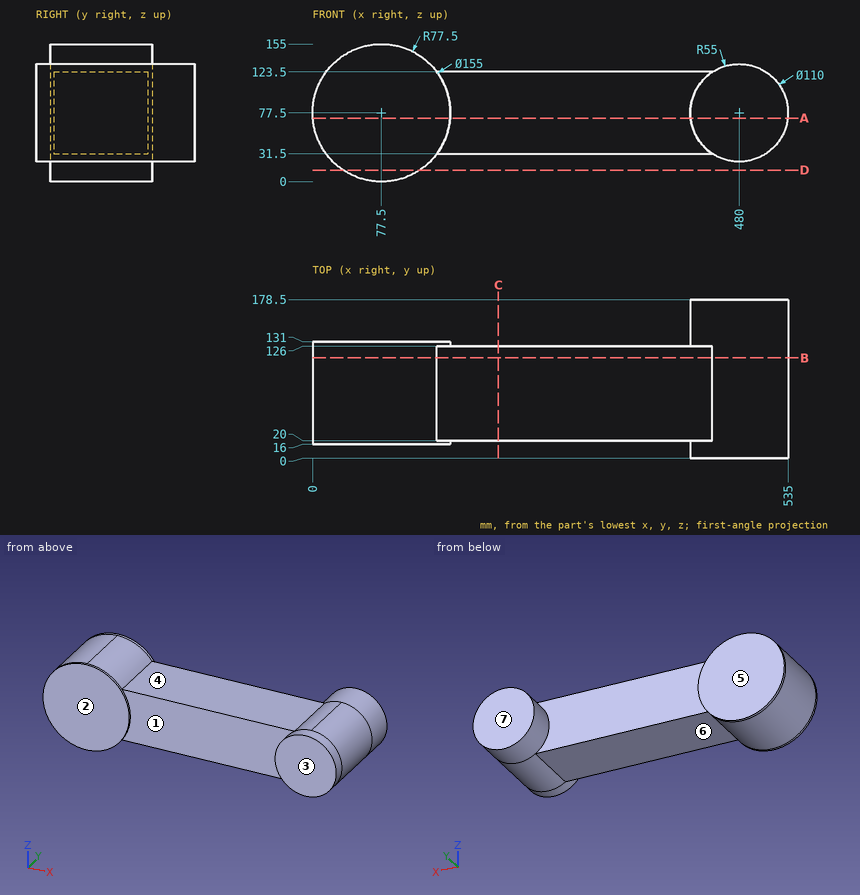
Job drawing, mm, ordinate dimensions from the low corner. One solid piece. A direction names the side the tool comes from. Give positions to 0.01 mm unless a question says otherwise; leave off trailing zeros. Loops run counter-clockwise (first coordinate to the right, second up) from the corner with the lowest first, then second, coordinate; pieces in that order, holes last. Notation, with made-up numbers: (-15.5, -8) - (35.5, -8) arc R27 ccw to (35.5, 25) - close; hole circle Ø3 at (36.5, 44). An arc over 180 degrees is marked (long way). Use one line per item in the form item = value.
(1) Cut at A-A (z = 71.5). Give the cut face in (x, y).
Determined:
outline = (0.23, 16) - (154.77, 16) - (154.77, 20) - (425.33, 20) - (425.33, 0) - (534.67, 0) - (534.67, 178.5) - (425.33, 178.5) - (425.33, 126) - (154.77, 126) - (154.77, 131) - (0.23, 131) - close
(2) Cut at C-C (x = 209). Give the cut face in (y, z), then the cut area to 3 significant figures.
Determined:
outline = (20, 31.5) - (126, 31.5) - (126, 123.5) - (20, 123.5) - close
area = 9,750 mm^2
(3) Drop flat-ended pins along their axis: P1, Ø12, axis at y = 68, z = 58.5, coming from the +X side; P2, Ø3, axis at y = 101.5, z = 64, coming from the -X side (1 decimal); P3, Ø12, axis at x = 395, y = 94, coming from the +Z side. Give the stop position or say it passes through.
Determined:
P1 = 533.44
P2 = 0.9
P3 = 123.5
(4) Pull direction X, two halves, no side cores. Call the marked faces 1 and 2: pulls with the +X half, pulls with the -X half, needs draft (parallel to the pull), parting line crosses it, or undercut.
Determined:
face_1 = undercut
face_2 = needs draft
(5) 3-axis set-ups, long thin cutter, end or side, ignore diameter. For the marked faces 3, 4, 5, 6 and 7: which of +Z, -Z, +X, -X, +Y, -Y reach the whole face in a straight line?
Determined:
face_3 = +Z, -Z, +X, -X, -Y
face_4 = +Z, +Y, -Y
face_5 = +Z, -Z, -X, +Y
face_6 = -Z, +Y, -Y
face_7 = +Z, -Z, +X, -X, +Y
(6) Cut at B-B (y = 113). Give the cut face in (x, z).
Determined:
outline = (139.87, 31.5) - (449.85, 31.5) arc R55 ccw (long way) to (449.85, 123.5) - (139.87, 123.5) arc R77.5 ccw (long way) to start
(7) Drill centre lines: L1, parallel to Y at x = 76.5, z = 141; L2, parallel to Y at x = 246, z = 74; L3, parallel to Z at x = 204, y = 104.5. Where is each one in solid material? Low to high.
Determined:
L1 = 16 to 131
L2 = 20 to 126
L3 = 31.5 to 123.5
(8) Cut at D-D (z = 13). Give the cut face in (x, y) (1 decimal).
Determined:
outline = (34.5, 16) - (120.5, 16) - (120.5, 131) - (34.5, 131) - close
